Autodesk Fusion 360 part; units mm, degrees
sketch "스케치1" plane through (0, 0, 0) normal (0, 0, 1) x (1, 0, 0)
  circle A0 centre (0, 0) radius 50
  circle A1 centre (125.1784, 0) radius 20
  line L0 (11.9829, 48.5429) -> (129.9716, 19.4171)
  line L1 (11.9829, -48.5429) -> (129.9716, -19.4171)
  circle A2 centre (0, 0) radius 40
  circle A3 centre (125.1784, 0) radius 12.5
  dimension "d1" = 100
  dimension "d2" = 40
  dimension "d3" = 80
  dimension "d4" = 25
extrude "돌출4" add sketch "스케치1" along normal blind 40 contours A0 makes body 1
extrude "돌출5" add sketch "스케치1" along normal blind 30 separate body contours A1 makes body 2
extrude "돌출6" add sketch "스케치1" along normal blind 15 contours A0 A1 L0 L1 bodies 1 2
Geometry check sheet. Reference: the model listing, model coordinates, mm. A direction names the side the tool comes from. Give positions to 0.01 mm unless a question says otherwise; leave off trailing zeros. Loops run counter-clockwise (first coordinate to the right, second up) from the corner with the lowest first, then second, coordinate; pieces in that order, holes last. Notation, with made-up numbers: M 9,34 L 26,34 A24 ccw 26,65 Z; hole C -32.5,-9.5 d2. An arc over 180 degrees is marked long. Answer as CSV lines item,"result".
Item 1: Release check for a two-part mould opening along X. For faces 4 (the flat face through (70, 1, 15)), 5 (the cylindrical face through (136.725, 4.788, 14.79)), 6 (the flat face through (70.151, -34.184, 7.395)), 7 (the flat face through (-22, 34, 40)) record: pulls with the +X half, pulls with the -X half, needs draft (parallel to the pull), parting line crosses it, or undercut.
Values:
face 4,"undercut"
face 5,"undercut"
face 6,"pulls with the +X half"
face 7,"needs draft"
Item 2: Cross-section at C-C on z = 26.5. Record the cut outline in (x, y), and give its area (3 significant figures).
Values:
outline,"C 0,0 d100; C 125.18,0 d40; hole C 0,0 d80; hole C 125.18,0 d25"
area,"3,590 mm²"
Item 3: Material ranges on line 1 (X direction, y = -5.5, z = 10); line 2 (X direction, y = -18, z = 17); line 3 (Y direction, x = 0, z = 34), recorded low to high.
Values:
line 1,"x = -49.7 to -39.62, 39.62 to 113.95, 136.4 to 144.41"
line 2,"x = -46.65 to -35.72, 35.72 to 46.65, 116.46 to 133.9"
line 3,"y = -50 to -40, 40 to 50"
Item 4: Depth check by flat-ended pin: P1, Ø5, axis at y = 4.5, z = 4, coming from the +X side; P2, Ø1, axis at y = 16.5, z = 35.5, coming from the -X side; P3, Ø3, axis at x = 34, z = 25, coming from the +Y side. Enter the tip coordinate at first touch or a pass-through.
Values:
P1,"stops at x = 145.08"
P2,"stops at x = -47.37"
P3,"stops at y = 38"
Item 5: Cross-section at A-A on y = 0. Record the cut outline in (x, z).
Values:
outline,"M -50,0 L -40,0 L -40,40 L -50,40 Z; M 40,0 L 112.68,0 L 112.68,30 L 105.18,30 L 105.18,15 L 50,15 L 50,40 L 40,40 Z; M 137.68,0 L 145.18,0 L 145.18,30 L 137.68,30 Z"
Item 6: Access from +Z, -Z, +X, -X, +Y, -Y to the whole of each face (thin tool, end or side, straight path). Record for faces 1 (the cylindrical face through (144.255, -6.007, 18.123)), 2 (the flat face through (46, 1, 0)), 3 (the flat face through (116, -9, 30)).
Values:
face 1,"+Z"
face 2,"-Z, +X, -X, +Y, -Y"
face 3,"+Z, +X, +Y, -Y"
Item 7: Cross-section at D-D on y = -27. Record the cut outline in (x, z).
Values:
outline,"M -42.08,0 L -29.51,0 L -29.51,40 L -42.08,40 Z; M 29.51,0 L 99.25,0 L 99.25,15 L 42.08,15 L 42.08,40 L 29.51,40 Z"
Item 8: Cross-section at B-B on x = 0. Record the cut outline in (y, z).
Values:
outline,"M -50,0 L -40,0 L -40,40 L -50,40 Z; M 40,0 L 50,0 L 50,40 L 40,40 Z"
